```python
from build123d import *

# Parameters (mm, degrees)
F1_DEPTH = 60.96


with BuildPart() as f1:
    # F0 (on Top) → F1 (new body)
    with BuildSketch(Plane.XY):
        Polygon((1066.8, 0), (762, 304.8), (-304.8, 304.8), (-762, 0), (-1066.8, 0), (-1066.8, -304.8), (1066.8, -304.8), align=None)
    extrude(amount=-F1_DEPTH)


solid = f1.part
```
Geometry check sheet. Reference: the model listing, model coordinates, mm. A direction names the side the tool comes from. Coordinates: 2 decimals unless noted, no trailing zeros. Order: outer loops, then holes, each group sorted by start corner. A loop starts at its lowest first (then second) coordinate and runs counter-clockwise, first axis right, second up. Notation, with made-up numbers: (-24, -16) - (4, -16) arc R10 cw to (4, 2) - close; hole circle Ø1 at (24, 49.5). An arc over 180 degrees is marked (long way). Answer in a Markdown table with one row per item. Add a question column.
1. Access from +Z, -Z, +X, -X, +Y, -Y to the whole of each face (thin tool, end or side, straight path). Record for faces 1 (the face through (-15, -304.8, -30)), 2 (the face through (-912, 0, -30)).
2. Section check A-A (z = -26). Enter the section's corners in (x, y), plus the area to 3 significant figures.
3. Gauge pin test, flat ends, axial feed: pin 1 Ø4 at (y, z) = (114.5, -7) entering from -X; pin 2 Ø2 at (x, z) = (-345, -38.5) entering from +Y. Record the tip position at first contact, or that the pin passes through.
4. Material ranges on L1, parallel to Y at x = -943, z = -31.5; L2, parallel to Y at x = 864.5, z = -48.5; L3, parallel to X at y = 13, z = -48, recorded low to high. Write a range as [from, to].
5. Section check C-C (x = -502). Enter the section's corners in (y, z), plus the area to 3 significant figures.
6. Section check B-B (y = 199.5). Enter the section's corners in (x, z), plus the area to 3 significant figures.
Data:
| question | item | result |
|---|---|---|
| 1 | face 1 | +Z, -Z, +X, -X, -Y |
| 1 | face 2 | +Z, -Z, -X, +Y |
| 2 | outline | (-1066.8, -304.8) - (1066.8, -304.8) - (1066.8, 0) - (762, 304.8) - (-304.8, 304.8) - (-762, 0) - (-1066.8, 0) - close |
| 2 | area | 1,090,000 mm² |
| 3 | pin 1 | stops at x = -593.25 |
| 3 | pin 2 | stops at y = 278.67 |
| 4 | L1 | y = [-304.8, 0] |
| 4 | L2 | y = [-304.8, 202.3] |
| 4 | L3 | x = [-742.5, 1053.8] |
| 5 | outline | (-304.8, -60.96) - (173.33, -60.96) - (173.33, 0) - (-304.8, 0) - close |
| 5 | area | 29,100 mm² |
| 6 | outline | (-462.75, -60.96) - (867.3, -60.96) - (867.3, 0) - (-462.75, 0) - close |
| 6 | area | 81,100 mm² |
